Here's how the part is built. I have some questions about the finished solid (model axes, mm). A direction names the side the tool comes from. Round coordinates to 2 decimals unless told otherwise and drop trailing zeros. Loops run counter-clockwise (first coordinate to the right, second up) from the corner with the lowest first, then second, coordinate; pieces in that order, holes last. Notation, with made-up numbers: (-32, 25.5) -> (-11, 25.5) arc R32 ccw to (-11, 51.5) -> close; hole circle Ø3 at (-6, 56.5). An arc over 180 degrees is marked (long way). Use one line per item in the form item = value. Start each with the question number.
Item 1: I'm going to push flat-ended pins straight in: pin 1 Ø1 at (y, z) = (-1, -58) entering from +X; pin 2 Ø4 at (x, z) = (10, -8.74) entering from -Y; pin 3 Ø10 at (x, y) = (45.5, -27.5) entering from -Z. Where does each tip first touch, or does it pass through?
Item 2: If we section it at C-C (x = 43): Write out the boundary of the cut face in (y, z).
Item 3: If I drill on L1, parallel to X at y = -0.45, z = -40.5; L2, parallel to Y at x = 57, z = -28; L3, parallel to Z at x = 22, y = -18, over which ranges is the centre line in solid material (lowest first)? Write a range as [from, to].
Item 4: If we section it at B-B (x = 53.5): Write out the boundary of the cut face in (y, z), then the cut area to 3 significant figures.
Item 5: Thinking about a two-plate mould opening in Z: for faces 3 (the face through (93.513, -0.986, -7.805)), 4 (the face through (50.7, -0.78, -3.823)), 5 (the face through (0, -1, -14)), which applies, released by +Z, released by -Z, zero draft, split by the parting line, or undercut?
Item 6: For faces 1 (the face through (49, -2, -28)), 2 (the face through (91.487, -0.986, -16.932)), which set-ups out of +Z, -Z, +X, -X, +Y, -Y let a thin tool reach every point of the face, with its end or its side?
Item 7: If we section it at D-D (y = -20.5): Write out the boundary of the cut face in (x, z).
Item 8: If we section it at A-A (z = -62.5): Write out the boundary of the cut face in (x, y), then the cut area to 3 significant figures.
```python
from build123d import *

# Parameters (mm, degrees)
SKETCH2_W                    = 100
SKETCH2_H                    = 85
BASE_FLANGE1_DEPTH           = 2
SKETCH15_R                   = 1.5
SKETCH15_W                   = 20
SKETCH15_H                   = 42
SKETCH15_W_2                 = 100
SKETCH15_H_2                 = 3
CUT_EXTRUDE2_DEPTH           = 10
EDGE_FLANGE3_STRIP_W         = 9.4732
EDGE_FLANGE3_STRIP_H         = 2
EDGE_FLANGE3_STRIP_CUT_DEPTH = 100
EDGE_FLANGE3_DEPTH           = 100
SKETCH23_W                   = 28
SKETCH23_H                   = 10
CUT_EXTRUDE3_DEPTH           = 10
SKETCH24_W                   = 28
SKETCH24_H                   = 3
TAB1_DEPTH                   = 2
SKETCH25_R                   = 1.5
CUT_EXTRUDE11_DEPTH          = 10
CUT_EXTRUDE7_DEPTH           = 10
CUT_EXTRUDE9_DEPTH           = 10
SKETCH34_R                   = 1.5
CUT_EXTRUDE10_DEPTH          = 10
SKETCH35_R                   = 3
SKETCH35_R_2                 = 3.5
CUT_EXTRUDE12_DEPTH          = 10


# Sheet-metal steps are written as plain solids
with BuildPart() as part:
    # Sketch2 → Base-Flange1 (new body)
    with BuildSketch(Plane(origin=(0, 0, 0), x_dir=(1, 0, 0), z_dir=(0, 1, 0))):
        with Locations((50, 42.5)):
            Rectangle(SKETCH2_W, SKETCH2_H)
    extrude(amount=-BASE_FLANGE1_DEPTH)

    # Sketch15 → Cut-Extrude2 (cut)
    with BuildSketch(Plane(origin=(0, 0, 0), x_dir=(1, 0, 0), z_dir=(0, 1, 0))):
        with Locations(Location((5, 8, 0), (0, 0, 270))):
            Circle(SKETCH15_R)
        with Locations(Location((5, 40.5, 0), (0, 0, 270))):
            Circle(SKETCH15_R)
        with Locations(Location((50, 80, 0), (0, 0, 270))):
            Circle(SKETCH15_R)
        with Locations(Location((95, 8, 0), (0, 0, 90))):
            Circle(SKETCH15_R)
        with Locations(Location((95, 40.5, 0), (0, 0, 90))):
            Circle(SKETCH15_R)
        with Locations((10, 64)):
            Rectangle(SKETCH15_W, SKETCH15_H)
        with Locations((90, 64)):
            Rectangle(SKETCH15_W, SKETCH15_H)
        with Locations((50, 1.5)):
            Rectangle(SKETCH15_W_2, SKETCH15_H_2)
    extrude(amount=-CUT_EXTRUDE2_DEPTH, mode=Mode.SUBTRACT)

    # Edge-Flange3 strip (across the edge) → Edge-Flange3 strip cut (cut)
    with BuildSketch(Plane(origin=(100, -2, -3), x_dir=(0, 0, -1), z_dir=(-1, 0, 0))):
        with Locations((-2, -1)):
            Rectangle(EDGE_FLANGE3_STRIP_W, EDGE_FLANGE3_STRIP_H)
    extrude(amount=EDGE_FLANGE3_STRIP_CUT_DEPTH, mode=Mode.SUBTRACT)

    # Edge-Flange3 section (across the edge) → Edge-Flange3 (add)
    with BuildSketch(Plane(origin=(100, -2, -3), x_dir=(0, 0, -1), z_dir=(-1, 0, 0))):
        with BuildLine():
            Line((0, 0.7366), (0, 38))
            Line((0, 38), (2, 38))
            Line((2, 38), (2, 0.7366))
            ThreePointArc((2, 0.7366), (2.215745145, 0.215745145), (2.7366, 0))
            Line((2.7366, 0), (2.7366, -2))
            ThreePointArc((2.7366, -2), (0.801531583, -1.198468417), (0, 0.7366))
        make_face()
    extrude(amount=EDGE_FLANGE3_DEPTH)

    # Sketch23 → Cut-Extrude3 (cut)
    with BuildSketch(Plane.XY.offset(-3)):
        with Locations((50, -35)):
            Rectangle(SKETCH23_W, SKETCH23_H)
    extrude(amount=-CUT_EXTRUDE3_DEPTH, mode=Mode.SUBTRACT)

    # Sketch24 → Tab1 (add)
    with BuildSketch(Plane.XY.offset(-3)):
        with Locations((50, -38.5)):
            Rectangle(SKETCH24_W, SKETCH24_H)
    extrude(amount=-TAB1_DEPTH)

    # Sketch25 → Cut-Extrude11 (cut)
    with BuildSketch(Plane(origin=(0, 0, 0), x_dir=(1, 0, 0), z_dir=(0, 1, 0))):
        with Locations(Location((43, 81, 0), (0, 0, 270))):
            Circle(SKETCH25_R)
        with Locations(Location((43, 22, 0), (0, 0, 270))):
            Circle(SKETCH25_R)
        with Locations(Location((9, 22, 0), (0, 0, 270))):
            Circle(SKETCH25_R)
        with Locations(Location((91, 22, 0), (0, 0, 90))):
            Circle(SKETCH25_R)
        with Locations(Location((57, 22, 0), (0, 0, 90))):
            Circle(SKETCH25_R)
        with Locations(Location((57, 81, 0), (0, 0, 90))):
            Circle(SKETCH25_R)
        with BuildLine():
            Line((37, 75), (63, 75))
            ThreePointArc((63, 75), (64.414213562, 74.414213562), (65, 73))
            Line((65, 73), (65, 37))
            ThreePointArc((65, 37), (64.414213562, 35.585786438), (63, 35))
            Line((63, 35), (37, 35))
            ThreePointArc((37, 35), (35.585786438, 35.585786438), (35, 37))
            Line((35, 37), (35, 73))
            ThreePointArc((35, 73), (35.585786438, 74.414213562), (37, 75))
        make_face()
    extrude(amount=-CUT_EXTRUDE11_DEPTH, mode=Mode.SUBTRACT)

    # Sketch28 → Cut-Extrude7 (cut)
    with BuildSketch(Plane(origin=(0, 0, 0), x_dir=(1, 0, 0), z_dir=(0, 1, 0))):
        with BuildLine():
            Line((34.5, 8.7366), (65.5, 8.7366))
            ThreePointArc((65.5, 8.7366), (66.914213562, 9.322386438), (67.5, 10.7366))
            Line((67.5, 10.7366), (67.5, 16.7366))
            ThreePointArc((67.5, 16.7366), (66.914213562, 18.150813562), (65.5, 18.7366))
            Line((65.5, 18.7366), (34.5, 18.7366))
            ThreePointArc((34.5, 18.7366), (33.085786438, 18.150813562), (32.5, 16.7366))
            Line((32.5, 16.7366), (32.5, 10.7366))
            ThreePointArc((32.5, 10.7366), (33.085786438, 9.322386438), (34.5, 8.7366))
        make_face()
    extrude(amount=-CUT_EXTRUDE7_DEPTH, mode=Mode.SUBTRACT)

    # Sketch33 → Cut-Extrude9 (cut)
    with BuildSketch(Plane.XY.offset(-3)):
        with BuildLine():
            Line((35, -4.7366), (37, -4.7366))
            ThreePointArc((37, -4.7366), (37.707106781, -5.029493219), (38, -5.7366))
            Line((38, -5.7366), (38, -6.7366))
            ThreePointArc((38, -6.7366), (37.707106781, -7.443706781), (37, -7.7366))
            Line((37, -7.7366), (35, -7.7366))
            ThreePointArc((35, -7.7366), (34.292893219, -7.443706781), (34, -6.7366))
            Line((34, -6.7366), (34, -5.7366))
            ThreePointArc((34, -5.7366), (34.292893219, -5.029493219), (35, -4.7366))
        make_face()
        with BuildLine():
            Line((35, -21.7366), (37, -21.7366))
            ThreePointArc((37, -21.7366), (37.707106781, -22.029493219), (38, -22.7366))
            Line((38, -22.7366), (38, -23.7366))
            ThreePointArc((38, -23.7366), (37.707106781, -24.443706781), (37, -24.7366))
            Line((37, -24.7366), (35, -24.7366))
            ThreePointArc((35, -24.7366), (34.292893219, -24.443706781), (34, -23.7366))
            Line((34, -23.7366), (34, -22.7366))
            ThreePointArc((34, -22.7366), (34.292893219, -22.029493219), (35, -21.7366))
        make_face()
        with BuildLine():
            Line((65, -24.7366), (63, -24.7366))
            ThreePointArc((63, -24.7366), (62.292893219, -24.443706781), (62, -23.7366))
            Line((62, -23.7366), (62, -22.7366))
            ThreePointArc((62, -22.7366), (62.292893219, -22.029493219), (63, -21.7366))
            Line((63, -21.7366), (65, -21.7366))
            ThreePointArc((65, -21.7366), (65.707106781, -22.029493219), (66, -22.7366))
            Line((66, -22.7366), (66, -23.7366))
            ThreePointArc((66, -23.7366), (65.707106781, -24.443706781), (65, -24.7366))
        make_face()
        with BuildLine():
            Line((65, -7.7366), (63, -7.7366))
            ThreePointArc((63, -7.7366), (62.292893219, -7.443706781), (62, -6.7366))
            Line((62, -6.7366), (62, -5.7366))
            ThreePointArc((62, -5.7366), (62.292893219, -5.029493219), (63, -4.7366))
            Line((63, -4.7366), (65, -4.7366))
            ThreePointArc((65, -4.7366), (65.707106781, -5.029493219), (66, -5.7366))
            Line((66, -5.7366), (66, -6.7366))
            ThreePointArc((66, -6.7366), (65.707106781, -7.443706781), (65, -7.7366))
        make_face()
    extrude(amount=-CUT_EXTRUDE9_DEPTH, mode=Mode.SUBTRACT)

    # Sketch34 → Cut-Extrude10 (cut)
    with BuildSketch(Plane(origin=(0, 0, 0), x_dir=(1, 0, 0), z_dir=(0, 1, 0))):
        with Locations(Location((10, 8.7366, 0), (0, 0, 270))):
            Circle(SKETCH34_R)
        with Locations(Location((90, 8.7366, 0), (0, 0, 270))):
            Circle(SKETCH34_R)
        with Locations(Location((14, 8.7366, 0), (0, 0, 270))):
            Circle(SKETCH34_R)
        with Locations(Location((14, 12.7366, 0), (0, 0, 270))):
            Circle(SKETCH34_R)
        with Locations(Location((10, 12.7366, 0), (0, 0, 270))):
            Circle(SKETCH34_R)
        with Locations(Location((90, 12.7366, 0), (0, 0, 270))):
            Circle(SKETCH34_R)
        with Locations(Location((90, 16.7366, 0), (0, 0, 270))):
            Circle(SKETCH34_R)
    extrude(amount=-CUT_EXTRUDE10_DEPTH, mode=Mode.SUBTRACT)

    # Sketch35 → Cut-Extrude12 (cut)
    with BuildSketch(Plane(origin=(0, 0, 0), x_dir=(1, 0, 0), z_dir=(0, 1, 0))):
        with Locations(Location((26.5, 13.7366, 0), (0, 0, 270))):
            Circle(SKETCH35_R)
        with Locations(Location((72.5, 13.7366, 0), (0, 0, 270))):
            Circle(SKETCH35_R_2)
        with Locations(Location((81.5, 13.7366, 0), (0, 0, 270))):
            Circle(SKETCH35_R_2)
    extrude(amount=-CUT_EXTRUDE12_DEPTH, mode=Mode.SUBTRACT)


solid = part.part
```
Values found:
q1.pin_1 = 80
q1.pin_2 = -2
q1.pin_3 = -5
q2.outline = (-40, -5) -> (-37, -5) -> (-37, -3) -> (-40, -3) -> close; (-30, -5) -> (-2.74, -5) arc R0.74 cw to (-2, -5.74) -> (-2, -8.74) -> (0, -8.74) -> (0, -5.74) arc R2.74 ccw to (-2.74, -3) -> (-30, -3) -> close; (-2, -85) -> (0, -85) -> (0, -82.5) -> (-2, -82.5) -> close; (-2, -79.5) -> (0, -79.5) -> (0, -75) -> (-2, -75) -> close; (-2, -35) -> (0, -35) -> (0, -23.5) -> (-2, -23.5) -> close; (-2, -20.5) -> (0, -20.5) -> (0, -18.74) -> (-2, -18.74) -> close
q3.L1 = [0, 3.5], [6.5, 35], [65, 93.5], [96.5, 100]
q3.L2 = [-2, 0]
q3.L3 = [-5, -3]
q4.outline = (-40, -5) -> (-37, -5) -> (-37, -3) -> (-40, -3) -> close; (-30, -5) -> (-2.74, -5) arc R0.74 cw to (-2, -5.74) -> (-2, -8.74) -> (0, -8.74) -> (0, -5.74) arc R2.74 ccw to (-2.74, -3) -> (-30, -3) -> close; (-2, -85) -> (0, -85) -> (0, -75) -> (-2, -75) -> close; (-2, -35) -> (0, -35) -> (0, -18.74) -> (-2, -18.74) -> close
q4.area = 125 mm2
q5.face_3 = undercut
q5.face_4 = released by +Z
q5.face_5 = zero draft
q6.face_1 = -Z, +X, -X, -Y
q6.face_2 = +Y, -Y
q7.outline = (0, -5) -> (100, -5) -> (100, -3) -> (0, -3) -> close
q8.outline = (20, -2) -> (35, -2) -> (35, 0) -> (20, 0) -> close; (65, -2) -> (80, -2) -> (80, 0) -> (65, 0) -> close
q8.area = 60.0 mm2
